from build123d import *

# Parameters (mm, degrees)
F0_R     = 5.715
F0_R_2   = 2.54
F1_DEPTH = 2.54
F2_DEPTH = 1.397


with BuildPart() as f1:
    # F0 (on Top) → F1 (new body, symmetric)
    with BuildSketch(Plane.XY):
        Circle(F0_R)
        Circle(F0_R_2, mode=Mode.SUBTRACT)
        Circle(F0_R_2)
    extrude(amount=F1_DEPTH, both=True)

    # F0 (on Top) → F2 (cut, symmetric)
    with BuildSketch(Plane.XY):
        Circle(F0_R)
        Circle(F0_R_2, mode=Mode.SUBTRACT)
    extrude(amount=F2_DEPTH, both=True, mode=Mode.SUBTRACT)


solid = f1.part
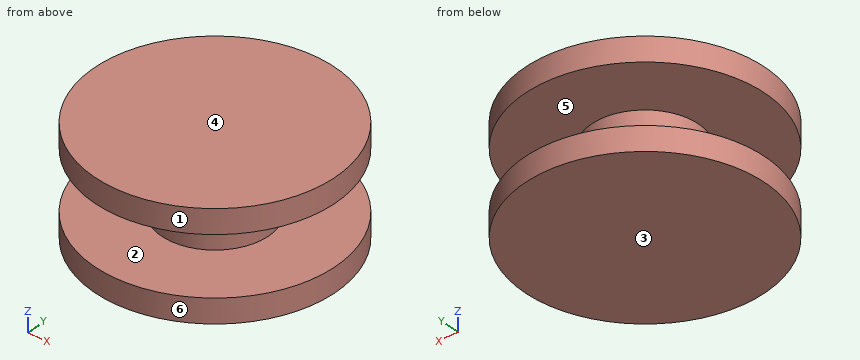
Can you work these out from the model? Positions are in its coordinate system, mm. Face numbers are marked on the shaded views. A direction names the side the tool comes from. Coordinates: 2 decimals unless noted, no trailing zeros. Order: outer loops, then holes, each group sorted by start corner. A loop starts at its lowest first (then second) coordinate and runs counter-clockwise, first axis right, second up. Notation, with made-up numbers: (8.25, 79.5) -> (23.25, 79.5) arc R25 cw to (23.25, 101.5) -> close; hole circle Ø11 at (16, 2). An arc over 180 degrees is marked (long way). Use one line per item in the form item = value.
Q1. Imagine slicing it at D-D, the plane z = -2. List the corners of the cut face in (x, y) for me (3 decimals), then the cut area to 3 significant figures.
From the geometry:
outline = circle Ø11.43 at (0, 0)
area = 103 mm²
Q2. I need wall thicknesses on L1, parallel to Z at x = -3.5, y = 0.25; L2, parallel to X at y = -4.25, z = -2; L3, parallel to Y at x = 0.5, z = 1.3. Which ranges of each line are inside material? Lowest first, please.
From the geometry:
L1 = -2.54 to -1.4, 1.4 to 2.54
L2 = -3.82 to 3.82
L3 = -2.49 to 2.49
Q3. We'd pull the mould along Z, two halves only. Please class the marked faces 1, 2, 3 and 4: released by +Z, released by -Z, zero draft, split by the parting line, or undercut.
From the geometry:
face_1 = zero draft
face_2 = undercut
face_3 = released by -Z
face_4 = released by +Z
Q4. Imagine slicing it at A-A, the plane y = -3.5. List the corners of the cut face in (x, z) for me, then the cut area to 3 significant figures.
From the geometry:
outline = (-4.52, -2.54) -> (4.52, -2.54) -> (4.52, -1.4) -> (-4.52, -1.4) -> close; (-4.52, 1.4) -> (4.52, 1.4) -> (4.52, 2.54) -> (-4.52, 2.54) -> close
area = 20.7 mm²
Q5. Imagine slicing it at B-B, the plane x = 0. List the corners of the cut face in (y, z) for me (3 decimals).
From the geometry:
outline = (-5.715, -2.54) -> (5.715, -2.54) -> (5.715, -1.397) -> (2.54, -1.397) -> (2.54, 1.397) -> (5.715, 1.397) -> (5.715, 2.54) -> (-5.715, 2.54) -> (-5.715, 1.397) -> (-2.54, 1.397) -> (-2.54, -1.397) -> (-5.715, -1.397) -> close
Q6. Which directions (+Z, -Z, +X, -X, +Y, -Y) give clear straight access to the entire face, cutting with the end or side of a thin tool? Please do the marked faces 5 and 6.
From the geometry:
face_5 = none
face_6 = +Z, -Z
